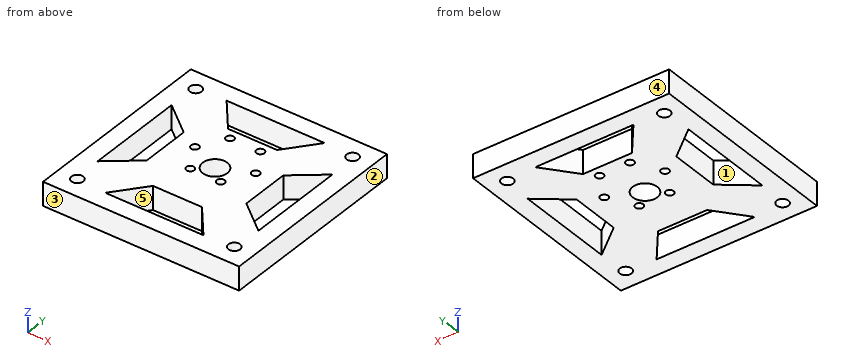
from build123d import *

# Parameters (mm, degrees)
ESQUISSE1_R             = 18.5
BOSS_EXTRU_1_DEPTH      = 12
ESQUISSE2_R             = 2
ENL_V_MAT_EXTRU_1_DEPTH = 13
ESQUISSE3_R             = 6.25
ENL_V_MAT_EXTRU_2_DEPTH = 13
ESQUISSE4_W             = 100
ESQUISSE4_H             = 100
ESQUISSE4_R             = 18.5
BOSS_EXTRU_2_DEPTH      = 12
ESQUISSE5_R             = 3
ENL_V_MAT_EXTRU_3_DEPTH = 12
ENL_V_MAT_EXTRU_4_DEPTH = 12


with BuildPart() as part:
    # Esquisse1 → Boss.-Extru.1 (new body)
    with BuildSketch(Plane.XY):
        Circle(ESQUISSE1_R)
    extrude(amount=BOSS_EXTRU_1_DEPTH)

    # Esquisse2 → Enlèv. mat.-Extru.1 (cut, through all)
    with BuildSketch(Plane.XY.offset(12)):
        with Locations((15.5, 0)):
            Circle(ESQUISSE2_R)
        with Locations((7.75, -13.423393759)):
            Circle(ESQUISSE2_R)
        with Locations((-7.75, -13.423393759)):
            Circle(ESQUISSE2_R)
        with Locations((-15.5, 0)):
            Circle(ESQUISSE2_R)
        with Locations((-7.75, 13.423393759)):
            Circle(ESQUISSE2_R)
        with Locations((7.75, 13.423393759)):
            Circle(ESQUISSE2_R)
    extrude(amount=-ENL_V_MAT_EXTRU_1_DEPTH, mode=Mode.SUBTRACT)

    # Esquisse3 → Enlèv. mat.-Extru.2 (cut, through all)
    with BuildSketch(Plane.XY.offset(12)):
        with Locations((0, -7)):
            Circle(ESQUISSE3_R)
    extrude(amount=-ENL_V_MAT_EXTRU_2_DEPTH, mode=Mode.SUBTRACT)

    # Esquisse4 → Boss.-Extru.2 (add)
    with BuildSketch(Plane.XY.offset(12)):
        with Locations((0, -7)):
            Rectangle(ESQUISSE4_W, ESQUISSE4_H)
        Circle(ESQUISSE4_R, mode=Mode.SUBTRACT)
    extrude(amount=-BOSS_EXTRU_2_DEPTH)

    # Esquisse5 → Enlèv. mat.-Extru.3 (cut)
    with BuildSketch(Plane.XY.offset(12)):
        with Locations((-40, 33)):
            Circle(ESQUISSE5_R)
        with Locations((40, 33)):
            Circle(ESQUISSE5_R)
        with Locations((40, -47)):
            Circle(ESQUISSE5_R)
        with Locations((-40, -47)):
            Circle(ESQUISSE5_R)
    extrude(amount=-ENL_V_MAT_EXTRU_3_DEPTH, mode=Mode.SUBTRACT)

    # Esquisse6 → Enlèv. mat.-Extru.4 (cut)
    with BuildSketch(Plane.XY.offset(12)):
        Polygon((-41, 18), (-41, -32), (-25.387505004, -19.5), (-25.387505004, 5.5), align=None)
        Polygon((12.5, 18.387505004), (25, 34), (-25, 34), (-12.5, 18.387505004), align=None)
        Polygon((25.387505004, -19.5), (41, -32), (41, 18), (25.387505004, 5.5), align=None)
        Polygon((-12.5, -32.387505004), (-25, -48), (25, -48), (12.5, -32.387505004), align=None)
    extrude(amount=-ENL_V_MAT_EXTRU_4_DEPTH, mode=Mode.SUBTRACT)


solid = part.part
Here's how the part is built. I have some questions about the finished solid (model axes, mm). Face numbers are marked on the shaded views. A direction names the side the tool comes from. Round coordinates to 2 decimals unless told otherwise and drop trailing zeros. Loops run counter-clockwise (first coordinate to the right, second up) from the corner with the lowest first, then second, coordinate; pieces in that order, holes last. Notation, with made-up numbers: (73, 41) - (117, 41) arc R22 ccw to (117, 49) - close; hole circle Ø8 at (26, -39). An arc over 180 degrees is marked (long way). One line per question, with ' | ' between items. Start each with the question number.
Q1. I want a section at D-D (z = 8). State how many separate pieces and enclosed holes the cut face has, then the cut area to 3 significant figures.
Q2. I want a section at B-B (y = -17.5). Write out the boundary of the cut face in (x, z).
Q3. We'd pull the mould along X, two halves only. Please class the marked faces 1, 2 and 3: +X half, -X half, draft (parallel to the pull), parting line (faces both ways), or undercut.
Q4. Please list where these lines run through material, in increasing order: line 1 (Y direction, x = 0, z = 6); line 2 (X direction, y = -2.5, z = 1); line 3 (Y direction, x = 7.75, z = 8.25). Write a range as [from, to].
Q5. Will this pin go through, and if not, where does the flat tip stop? pin 1 (6.5 mm diameter, centred on x = -15.5, y = 0, fed in from +Z).
Q6. I want a section at C-C (y = -35.5). Write out the boundary of the cut face in (x, z), then the cut area to 3 significant figures.
Q7. For the marked faces 4 and 5, which set-ups out of +Z, -Z, +X, -X, +Y, -Y let a thin tool reach every point of the face, with its end or its side?
Q8. I want a section at A-A (x = 0). Write out the boundary of the cut face in (y, z).
Response values:
1) separate pieces: 1 | enclosed holes: 15 | area: 7,350 mm²
2) outline: (-50, 0) - (-41, 0) - (-41, 12) - (-50, 12) - close; (-25.39, 0) - (25.39, 0) - (25.39, 12) - (-25.39, 12) - close; (41, 0) - (50, 0) - (50, 12) - (41, 12) - close
3) face 1: undercut | face 2: +X half | face 3: draft
4) line 1: y = [-57, -48], [-32.39, -13.25], [-0.75, 18.39], [34, 43] | line 2: x = [-50, -41], [-25.39, -4.34], [4.34, 25.39], [41, 50] | line 3: y = [-57, -48], [-32.39, -15.42], [-11.42, 11.42], [15.42, 18.39], [34, 43]
5) pin 1: stops at z = 12
6) outline: (-50, 0) - (-14.99, 0) - (-14.99, 12) - (-50, 12) - close; (14.99, 0) - (50, 0) - (50, 12) - (14.99, 12) - close | area: 840 mm²
7) face 4: +Z, -Z, +X, -X, +Y | face 5: +Z, -Z
8) outline: (-57, 0) - (-48, 0) - (-48, 12) - (-57, 12) - close; (-32.39, 0) - (-13.25, 0) - (-13.25, 12) - (-32.39, 12) - close; (-0.75, 0) - (18.39, 0) - (18.39, 12) - (-0.75, 12) - close; (34, 0) - (43, 0) - (43, 12) - (34, 12) - close
